Work out the finished part from the listing and answer in its coordinate system (mm). A direction names the side the tool comes from. Round coordinates to 2 decimals unless told otherwise and drop trailing zeros. Write each loop counter-clockwise with the first axis right and the second up, starting at its lowest first coordinate (ties: lowest second). Pieces come first, ordered by that corner, then holes. Notation, with made-up numbers: (17, 22.5) -> (25, 22.5) arc R32 cw to (25, 54.5) -> close; hole circle Ø7 at (88, 59). An arc over 180 degrees is marked (long way). Answer as a JSON object with one key per item and string values. Group by question number.
from build123d import *

# Parameters (mm, degrees)
F0_R     = 11.025
F0_R_2   = 5.5
F1_DEPTH = 2.5
F0_R_3   = 4.075
F2_DEPTH = 3
F3_DEPTH = 5.5


# Not quite as in the source:
# - a fillet or chamfer that OpenCascade refuses, or shapes differently, is made with other operations: its cross-section is extruded or revolved along the edge and cut away or added


with BuildPart() as f1:
    # F0 (on Top) → F1 (new body)
    with BuildSketch(Plane.XY):
        Circle(F0_R)
        Circle(F0_R_2, mode=Mode.SUBTRACT)
    extrude(amount=F1_DEPTH)

    # F0 (on Top) → F2 (join)
    with BuildSketch(Plane.XY):
        Circle(F0_R_2)
        Circle(F0_R_3, mode=Mode.SUBTRACT)
    extrude(amount=F2_DEPTH)

    # F0 (on Top) → F3 (join)
    with BuildSketch(Plane.XY):
        Circle(F0_R_3)
    extrude(amount=F3_DEPTH)

    # F4: fillet of radius 3.5 on 1 edges, made by hand

    # F4_s1 → F4_t2 (revolve, cut)
    with BuildSketch(Plane.XZ):
        with BuildLine():
            ThreePointArc((11.025, 2.5), (9.7625481001, 0.6937569599), (7.6708980338, 0))
            Line((7.6708980338, 0), (11.025, 0))
            Line((11.025, 0), (11.025, 2.5))
        make_face()
    revolve(axis=Axis((0, 0, 0), (0, 0, 1)), mode=Mode.SUBTRACT)


solid = f1.part
1) Each of these flat-tipped pins is pushed along its axis until it touches: P1, Ø2, axis at x = 7, z = 3, coming from the -Y side; P2, Ø1, axis at x = -1.5, z = 0.5, coming from the -Y side; P3, Ø3, axis at y = 7.5, z = 1, coming from the +X side (3 decimals). Where does it stop, or does it pass through?
2) A tool of negligible diameter and unlimited length cuts with its end or side. For faces 1 (the face through (0, 0, 5.5)), 2 (the face through (-5, 3, 2.5)), from which of +Z, -Z, +X, -X, +Y, -Y can it reach the whole face along a straight path? Write none if from no direction.
3) A cutting plane is placed at C-C on z = 0.8. Determine the outline of the cut face in (x, y).
4) Straight lines are drawn through the part: L1, parallel to Z at x = -7.75, y = -0.75; L2, parallel to Z at x = 1.5, y = -5; L3, parallel to Y at x = 3.75, z = 4.45. For each, find the intervals that lie inside material, in ascending order.
5) A cutting plane is placed at A-A on x = 0. Determine the outline of the cut face in (y, z) (3 decimals), plus the area to 3 significant figures.
Established:
{
 "1": {"P1": "stops at y = -9.16", "P2": "stops at y = -10.01", "P3": "stops at x = 8.755"},
 "2": {"face 1": "+Z, +X, -X, +Y, -Y", "face 2": "+Z"},
 "3": {"outline": "circle Ø19.8 at (0, 0)"},
 "4": {"L1": "z = 0 to 2.5", "L2": "z = 0 to 3", "L3": "y = -1.59 to 1.59"},
 "5": {"outline": "(-11.025, 2.5) arc R3.5 ccw to (-7.671, 0) -> (7.671, 0) arc R3.5 ccw to (11.025, 2.5) -> (5.5, 2.5) -> (5.5, 3) -> (4.075, 3) -> (4.075, 5.5) -> (-4.075, 5.5) -> (-4.075, 3) -> (-5.5, 3) -> (-5.5, 2.5) -> close", "area": "76.6 mm²"}
}
